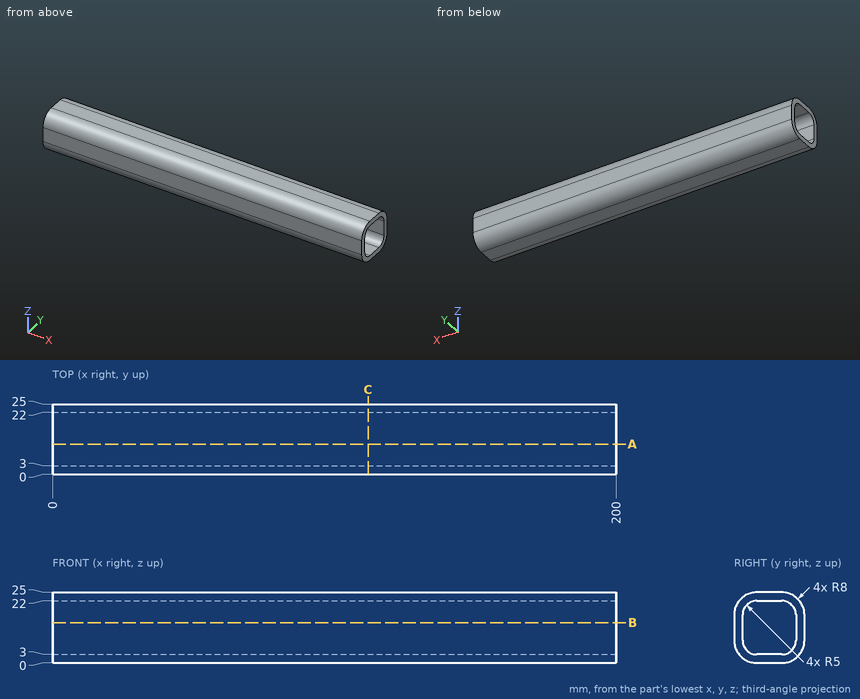
Print and shaded views of the part. All mm, measured from the part's lowest x, y and z. Round coordinates to 2 decimals unless told otherwise and drop trailing zeros. Write each loop counter-clockwise with the first axis right and the second up, starting at its lowest first coordinate (ties: lowest second). Pieces come first, ordered by that corner, then holes.
Item 1: Drop flat-ended pins along their axis: pin 1 Ø3 at (x, z) = (26, 6) entering from +Y; pin 2 Ø6 at (x, z) = (83, 4) entering from -Y. Give the stop position or say it passes through.
Results:
pin 1: stops at y = 24.98
pin 2: stops at y = 0.06
Item 2: Cut at A-A, the plane y = 10.75. Give the cut face in (x, z), plus the area to 3 significant figures.
Results:
outline: (0, 0) - (200, 0) - (200, 3) - (0, 3) - close; (0, 22) - (200, 22) - (200, 25) - (0, 25) - close
area: 1,200 mm2
Item 3: Probe L1, parallel to Z at x = 147, y = 14; L2, parallel to Y at x = 46, z = 19. List the from-to ranges inside material, lowest first.
Results:
L1: z = 0 to 3, 22 to 25
L2: y = 0.25 to 3.42, 21.58 to 24.75
Item 4: Cut at C-C, the plane x = 112. Give the cut face in (y, z).
Results:
outline: (0, 8) arc R8 ccw to (8, 0) - (17, 0) arc R8 ccw to (25, 8) - (25, 17) arc R8 ccw to (17, 25) - (8, 25) arc R8 ccw to (0, 17) - close; hole (3, 8) arc R5 ccw to (8, 3) - (17, 3) arc R5 ccw to (22, 8) - (22, 17) arc R5 ccw to (17, 22) - (8, 22) arc R5 ccw to (3, 17) - close
